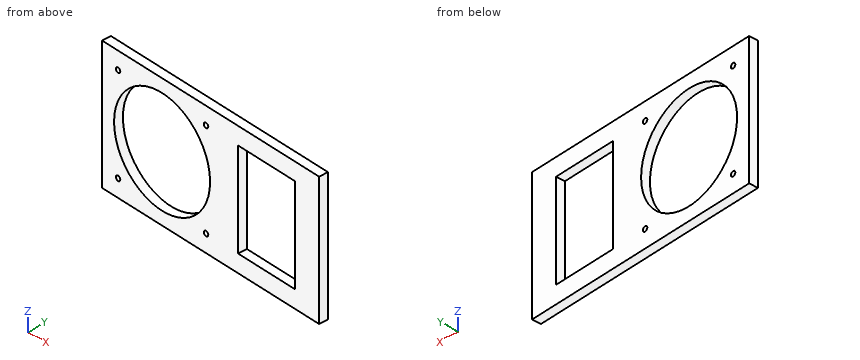
from build123d import *

# Parameters (mm, degrees)
BOSS_EXTRUDE1_DEPTH = 95.25
SKETCH3_R           = 38.1
CUT_EXTRUDE1_DEPTH  = 22.306729365
SKETCH4_R           = 1.75
CUT_EXTRUDE2_DEPTH  = 22.306729365
SKETCH5_W           = 45.264743179
SKETCH5_H           = 69.85
CUT_EXTRUDE3_DEPTH  = 22.306729365


with BuildPart() as part:
    # Sketch2 → Boss-Extrude1 (new body)
    with BuildSketch(Plane.XY):
        Polygon((-137.563755829, 331.29726238), (-138.117194795, 324.971426047), (33.492029028, 309.957564406), (34.045467994, 316.283400739), align=None)
    extrude(amount=BOSS_EXTRUDE1_DEPTH)

    # Sketch3 → Cut-Extrude1 (cut, through all)
    with BuildSketch(Plane(origin=(27.719631662, 316.836839705, 0), x_dir=(0.996194698, -0.087155743, 0), z_dir=(0.087155743, 0.996194698, 0))):
        with Locations((-118.289743179, -47.625)):
            Circle(SKETCH3_R)
    extrude(amount=-CUT_EXTRUDE1_DEPTH, mode=Mode.SUBTRACT)

    # Sketch4 → Cut-Extrude2 (cut, through all)
    with BuildSketch(Plane(origin=(27.719631662, 316.836839705, 0), x_dir=(0.996194698, -0.087155743, 0), z_dir=(0.087155743, 0.996194698, 0))):
        with Locations((-153.214743179, -12.7)):
            Circle(SKETCH4_R)
        with Locations((-153.214743179, -82.55)):
            Circle(SKETCH4_R)
        with Locations((-83.364743179, -82.55)):
            Circle(SKETCH4_R)
        with Locations((-83.364743179, -12.7)):
            Circle(SKETCH4_R)
    extrude(amount=-CUT_EXTRUDE2_DEPTH, mode=Mode.SUBTRACT)

    # Sketch5 → Cut-Extrude3 (cut, through all)
    with BuildSketch(Plane(origin=(27.719631662, 316.836839705, 0), x_dir=(0.996194698, -0.087155743, 0), z_dir=(0.087155743, 0.996194698, 0))):
        with Locations((-35.332371589, -47.625)):
            Rectangle(SKETCH5_W, SKETCH5_H)
    extrude(amount=-CUT_EXTRUDE3_DEPTH, mode=Mode.SUBTRACT)


solid = part.part
Check sheet for the modelled part. Datum: model origin and axes. Units: mm. Round coordinates to 2 decimals unless told otherwise and drop trailing zeros. Loops run counter-clockwise (first coordinate to the right, second up) from the corner with the lowest first, then second, coordinate; pieces in that order, holes last. Notation, with made-up numbers: M 74.25,33.25 L 133.25,33.25 A26 ccw 133.25,66.25 Z; hole C 74,-39.5 d1. An arc over 180 degrees is marked long. One line per question, with ' | ' between items. Start each with the question number.
Item 1: Section check B-B (x = -21). Record the boundary of the cut face in (y, z) (3 decimals).
Item 2: Scan lines: probe 1 along Z at (x, y) = (-90, 323.5); probe 2 along Z at (x, y) = (-11.5, 319.25); probe 3 along X at (y, z) = (315, 25). Record each from-to range of solid material in increasing order.
Item 3: Gauge pin test, flat ends, axial feed: pin 1 Ø8 at (x, z) = (12.5, 57) entering from -Y; pin 2 Ø6 at (x, y) = (4, 315.5) entering from -Z; pin 3 Ø4 at (x, z) = (-5.5, 15.5) entering from -Y. Record the tip position at first contact, or that the pin passes through.
Item 4: Section check C-C (z = 73.5). Record the boundary of the cut face in (x, y).
Item 5: Section check A-A (z = 59.5). Record the boundary of the cut face in (x, y), and give its area (3 significant figures).
Item 6: Section check D-D (y = 320). State how many separate pieces and enclosed holes the cut face has, and give its area (3 significant figures).
Worked out:
1) outline: M 314.725,0 L 321.099,0 L 321.099,12.7 L 314.725,12.7 Z; M 314.725,82.55 L 321.099,82.55 L 321.099,95.25 L 314.725,95.25 Z
2) probe 1: 0 to 9.53, 85.72 to 95.25 | probe 2: 0 to 12.7, 82.55 to 95.25 | probe 3: 14.81 to 33.93
3) pin 1: y = 311.44 | pin 2: z = 0 | pin 3: through
4) outline: M -138.12,324.97 L -118.53,323.26 L -117.98,329.58 L -137.56,331.3 Z; M -62.81,318.38 L -30.58,315.56 L -30.02,321.89 L -62.26,324.71 Z; M 14.51,311.62 L 33.49,309.96 L 34.05,316.28 L 15.07,317.94 Z
5) outline: M -138.12,324.97 L -126.74,323.98 L -126.18,330.3 L -137.56,331.3 Z; M -54.61,317.67 L -30.58,315.56 L -30.02,321.89 L -54.06,323.99 Z; M 14.51,311.62 L 33.49,309.96 L 34.05,316.28 L 15.07,317.94 Z | area: 347 mm^2
6) separate pieces: 1 | enclosed holes: 2 | area: 3,820 mm^2
